Job drawing, mm, ordinate dimensions from the low corner. One solid piece. Coordinates: 2 decimals unless noted, no trailing zeros. Write each loop counter-clockwise with the first axis right and the second up, starting at its lowest first coordinate (ties: lowest second). Pieces come first, ordered by that corner, then holes. Notation, with made-up numbers: (21.25, 13) - (47.25, 13) arc R23 cw to (47.25, 40) - close; hole circle Ø5 at (19.5, -16). An arc over 180 degrees is marked (long way). Put each result on its own line as item: value. Start each with the question number.
1. Saw through at A-A, the plane x = 5.08. Write the cut outline in (y, z) (1 decimal), plus the area to 3 significant figures.
2. Drop flat-ended pins along their axis: P1, Ø5, axis at x = 5.08, y = 5.08, coming from the +Z side; P2, Ø1.5, axis at x = 42, y = 14.5, coming from the -Z side. Give the stop position or say it passes through.
3. Saw through at B-B, the plane y = 5.08. Write the cut outline in (x, z) (1 decimal).
4. Saw through at C-C, the plane y = 17. Write the cut outline in (x, z).
5. Drill centre lines: L1, parallel to Y at x = 5.08, z = 0.9 (1 decimal); L2, parallel to X at y = 5, z = 1.25 (1 decimal); L3, parallel to X at y = 16.75, z = 1.3. Where is each one in solid material? Low to high. Write a range as from..to.
6. Saw through at D-D, the plane z = 0.3. Give the number of separate pieces and of enclosed holes in the cut face, plus the area to 3 significant figures.
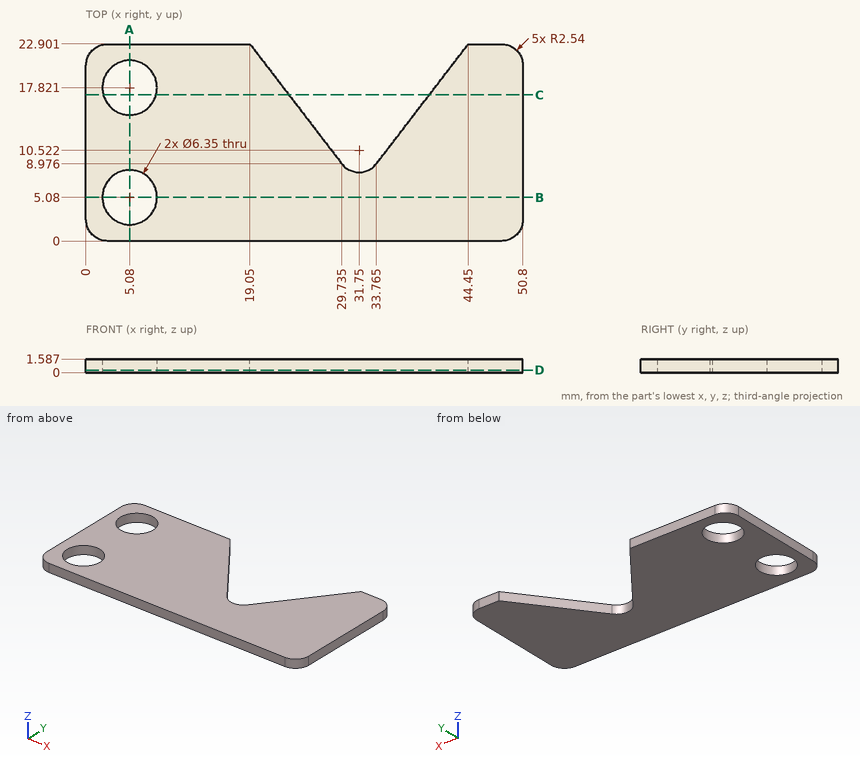
Final values:
1. outline: (0, 0) - (1.9, 0) - (1.9, 1.6) - (0, 1.6) - close; (8.3, 0) - (14.6, 0) - (14.6, 1.6) - (8.3, 1.6) - close; (21, 0) - (22.9, 0) - (22.9, 1.6) - (21, 1.6) - close
1. area: 16.2 mm²
2. P1: passes through
2. P2: stops at z = 0
3. outline: (0, 0) - (1.9, 0) - (1.9, 1.6) - (0, 1.6) - close; (8.3, 0) - (50.8, 0) - (50.8, 1.6) - (8.3, 1.6) - close
4. outline: (0, 0) - (2.01, 0) - (2.01, 1.59) - (0, 1.59) - close; (8.15, 0) - (23.58, 0) - (23.58, 1.59) - (8.15, 1.59) - close; (39.92, 0) - (50.8, 0) - (50.8, 1.59) - (39.92, 1.59) - close
5. L1: y = 0..1.9, 8.3..14.6, 21..22.9
5. L2: x = 0..1.9, 8.3..50.8
5. L3: x = 0..2.09, 8.07..23.77, 39.73..50.8
6. separate pieces: 1
6. enclosed holes: 2
6. area: 887 mm²
